Can you work these out from the model? Positions are in its coordinate system, mm. Face numbers are marked on the shaded views. A direction names the side the tool comes from. Give positions to 0.01 mm unless a question says otherwise; leave off trailing zeros. Loops run counter-clockwise (first coordinate to the right, second up) from the corner with the lowest first, then second, coordinate; pieces in that order, holes last. Notation, with made-up numbers: (48, -31.75) - (59, -31.75) arc R17 cw to (59, -15.75) - close; hole circle Ø2 at (42, -32). An arc over 180 degrees is marked (long way). Answer in a Markdown table with one row per item.
from build123d import *

# Parameters (mm, degrees)
SZKIC1_R                    = 33
DODANIE_WYCI_GNI_CIE1_DEPTH = 25
SZKIC2_R                    = 36
DODANIE_WYCI_GNI_CIE2_DEPTH = 2.5
SZKIC4_R                    = 31.5
DODANIE_WYCI_GNI_CIE3_DEPTH = 25
SZKIC11_R                   = 28.35
WYTNIJ_WYCI_GNI_CIE5_DEPTH  = 27.5
SZKIC12_R                   = 25
WYTNIJ_WYCI_GNI_CIE6_DEPTH  = 27.5
WYTNIJ_WYCI_GNI_CIE7_START  = -8
SZKIC13_R                   = 28.35
WYTNIJ_WYCI_GNI_CIE7_DEPTH  = 8
SFAZOWANIE1_SIZE            = 1
SFAZOWANIE2_SIZE            = 1
WYTNIJ_WYCI_GNI_CIE11_DEPTH = 25
ZAOKR_GLENIE1_R             = 10


with BuildPart() as part:
    # Szkic1 → Dodanie-wyciągnięcie1 (new body)
    with BuildSketch(Plane.XY):
        Circle(SZKIC1_R)
    extrude(amount=-DODANIE_WYCI_GNI_CIE1_DEPTH)

    # Szkic2 → Dodanie-wyciągnięcie2 (add)
    with BuildSketch(Plane(origin=(0, 0, -25), x_dir=(-1, 0, 0), z_dir=(0, 0, -1))):
        Circle(SZKIC2_R)
    extrude(amount=DODANIE_WYCI_GNI_CIE2_DEPTH)

    # Szkic4 → Dodanie-wyciągnięcie3 (add)
    with BuildSketch(Plane(origin=(0, 0, -27.5), x_dir=(-1, 0, 0), z_dir=(0, 0, -1))):
        Circle(SZKIC4_R)
    extrude(amount=DODANIE_WYCI_GNI_CIE3_DEPTH)

    # Szkic11 → Wytnij-wyciągnięcie5 (cut)
    with BuildSketch(Plane.XY):
        Circle(SZKIC11_R)
    extrude(amount=-WYTNIJ_WYCI_GNI_CIE5_DEPTH, mode=Mode.SUBTRACT)

    # Szkic12 → Wytnij-wyciągnięcie6 (cut)
    with BuildSketch(Plane.XY.offset(-27.5)):
        Circle(SZKIC12_R)
    extrude(amount=-WYTNIJ_WYCI_GNI_CIE6_DEPTH, mode=Mode.SUBTRACT)

    # Szkic13 → Wytnij-wyciągnięcie7 (cut)
    with BuildSketch(Plane(origin=(0, 0, -52.5), x_dir=(-1, 0, 0), z_dir=(0, 0, -1)).offset(WYTNIJ_WYCI_GNI_CIE7_START)):
        with Locations(Location((0, 0, 0), (0, 0, 180))):
            Circle(SZKIC13_R)
    extrude(amount=WYTNIJ_WYCI_GNI_CIE7_DEPTH, mode=Mode.SUBTRACT)

    # Sfazowanie1
    sfazowanie1_edges = [part.edges().sort_by_distance(p)[0] for p in [
        (-28.35, 0, 0),
    ]]
    chamfer(sfazowanie1_edges, length=SFAZOWANIE1_SIZE)

    # Sfazowanie2
    sfazowanie2_edges = [part.edges().sort_by_distance(p)[0] for p in [
        (-28.35, 0, -52.5),
    ]]
    chamfer(sfazowanie2_edges, length=SFAZOWANIE2_SIZE)

    # Szkic10 → Wytnij-wyciągnięcie11 (cut)
    with BuildSketch(Plane.XY):
        with BuildLine():
            Line((-23.334523779, -23.334523779), (-33, 0))
            ThreePointArc((-33, 0), (-30.488024573, -12.628553268), (-23.334523779, -23.334523779))
        make_face()
        with BuildLine():
            Line((-33, 0), (-23.334523779, 23.334523779))
            ThreePointArc((-23.334523779, 23.334523779), (-30.488024573, 12.628553268), (-33, 0))
        make_face()
        with BuildLine():
            Line((0, -33), (-23.334523779, -23.334523779))
            ThreePointArc((-23.334523779, -23.334523779), (-12.628553268, -30.488024573), (0, -33))
        make_face()
        with BuildLine():
            ThreePointArc((0, -33), (12.628553268, -30.488024573), (23.334523779, -23.334523779))
            Line((23.334523779, -23.334523779), (0, -33))
        make_face()
        with BuildLine():
            ThreePointArc((23.334523779, -23.334523779), (30.488024573, -12.628553268), (33, 0))
            Line((33, 0), (23.334523779, -23.334523779))
        make_face()
        with BuildLine():
            ThreePointArc((33, 0), (30.488024573, 12.628553268), (23.334523779, 23.334523779))
            Line((23.334523779, 23.334523779), (33, 0))
        make_face()
        with BuildLine():
            ThreePointArc((23.334523779, 23.334523779), (12.628553268, 30.488024573), (0, 33))
            Line((0, 33), (23.334523779, 23.334523779))
        make_face()
        with BuildLine():
            Line((-23.334523779, 23.334523779), (0, 33))
            ThreePointArc((0, 33), (-12.628553268, 30.488024573), (-23.334523779, 23.334523779))
        make_face()
    extrude(amount=-WYTNIJ_WYCI_GNI_CIE11_DEPTH, mode=Mode.SUBTRACT)

    # Szkic14 → Wycięcie-obrót3 (revolve, cut)
    with BuildSketch(Plane(origin=(0, 0, 0), x_dir=(0, 0, -1), z_dir=(1, 0, 0)), mode=Mode.PRIVATE) as wyci_cie_obr_t3_sk:
        Polygon((0, 33), (0, 31), (3, 33), align=None)
    revolve(wyci_cie_obr_t3_sk.sketch.rotate(Axis((0, 0, 0), (0, 0, -1)), 270), axis=Axis((0, 0, 0), (0, 0, -1)), mode=Mode.SUBTRACT)

    # Zaokrąglenie1
    zaokr_glenie1_edges = [part.edges().sort_by_distance(p)[0] for p in [
        (-23.334523779, 23.334523779, -14),
        (0, 33, -14),
        (23.334523779, 23.334523779, -14),
        (33, 0, -14),
        (23.334523779, -23.334523779, -14),
        (0, -33, -14),
        (-23.334523779, -23.334523779, -14),
        (-33, 0, -14),
    ]]
    fillet(zaokr_glenie1_edges, radius=ZAOKR_GLENIE1_R)


solid = part.part
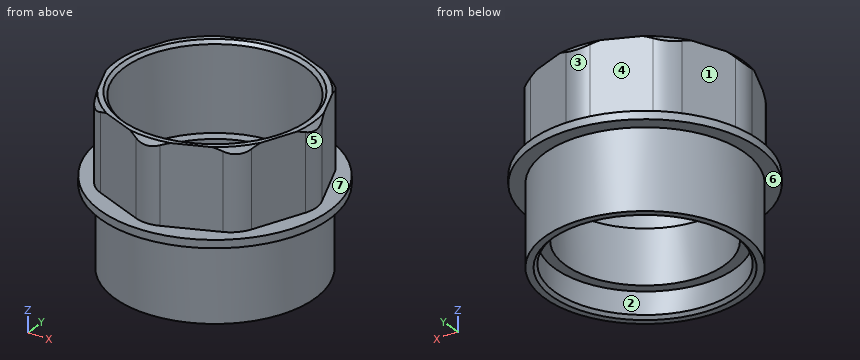
Q1. Imagine slicing it at C-C, the plane z = -11.5. Write out the boundary of the cut face in (x, y), and give its area (3 significant figures).
Checked values:
| item | result |
|---|---|
| outline | (-31.41, -3.83) - (-24.92, -19.51) arc R10 ccw to (-19.51, -24.92) - (-3.83, -31.41) arc R10 ccw to (3.83, -31.41) - (19.51, -24.92) arc R10 ccw to (24.92, -19.51) - (31.41, -3.83) arc R10 ccw to (31.41, 3.83) - (24.92, 19.51) arc R10 ccw to (19.51, 24.92) - (3.83, 31.41) arc R10 ccw to (-3.83, 31.41) - (-19.51, 24.92) arc R10 ccw to (-24.92, 19.51) - (-31.41, 3.83) arc R10 ccw to start; hole circle Ø56.7 at (0, 0) |
| area | 538 mm² |
Q2. For pin 1 (6 mm diameter, centred on x = -19, z = -45.5, fed in from -Y); pin 2 (5 mm diameter, centred on x = -26, z = -42.5, fed in from -Y); pin 3 (5 mm diameter, centred on x = -13.5, z = -10, fed in from -Y); pin 4 (21.5 mm diameter, centred on x = 6.5, y = 5.5, fed in from +Z), each with a flat end and sliding along its axis, tell me the tip position at first contact or that it passes through.
Checked values:
| item | result |
|---|---|
| pin 1 | stops at y = -27.13 |
| pin 2 | stops at y = -20.98 |
| pin 3 | stops at y = -28.44 |
| pin 4 | passes through |
Q3. If I drill on line 1 (Y direction, x = 0, z = -49.5); line 2 (Y direction, x = 0, z = -7); line 3 (Z direction, x = -15.5, y = -28), over which ranges is the centre line in solid material (lowest first)? Write a range as [from, to].
Checked values:
| item | result |
|---|---|
| line 1 | y = [-31.5, -28.35], [28.35, 31.5] |
| line 2 | y = [-32.18, -28.35], [28.35, 32.18] |
| line 3 | z = [-27.5, -25] |
Q4. On a 3-axis mill with a long thin cutter (end or side, diameter ignored), from which of +Z, -Z, +X, -X, +Y, -Y can I reach the whole of each face in a straight line? I mean the marked faces 4, 5, 6 and 7. Say none if no direction works.
Checked values:
| item | result |
|---|---|
| face 4 | +Z, -X, +Y |
| face 5 | +Z, +X |
| face 6 | -Z |
| face 7 | +Z |
Q5. Imagine slicing it at D-D, the plane z = -37.5. Write out the boundary of the cut face in (x, y), and give its area (3 significant figures).
Checked values:
| item | result |
|---|---|
| outline | circle Ø63 at (0, 0); hole circle Ø50 at (0, 0) |
| area | 1,150 mm² |
Q6. If we mould it in two halves opening along X, with no side actions, what happens to the marked faces 1, 2 and 3? For each: released by +X, released by -X, zero draft, split by the parting line, or undercut.
Checked values:
| item | result |
|---|---|
| face 1 | released by -X |
| face 2 | undercut |
| face 3 | split by the parting line |
